from build123d import *

# Parameters (mm, degrees)
SKETCH1_W           = 177.8
SKETCH1_H           = 177.8
BOSS_EXTRUDE1_DEPTH = 12.7
SKETCH2_R           = 3.175
CUT_EXTRUDE3_DEPTH  = 13.7
SKETCH4_W           = 12.7
SKETCH4_H           = 25.4
CUT_EXTRUDE4_DEPTH  = 13.7


with BuildPart() as part:
    # Sketch1 → Boss-Extrude1 (new body)
    with BuildSketch(Plane.XY):
        with Locations((88.9, -88.9)):
            Rectangle(SKETCH1_W, SKETCH1_H)
    extrude(amount=BOSS_EXTRUDE1_DEPTH)

    # Sketch2 → Cut-Extrude3 (cut, through all)
    with BuildSketch(Plane.XY.offset(12.7)):
        with Locations((104.14, -76.2)):
            Circle(SKETCH2_R)
    extrude(amount=-CUT_EXTRUDE3_DEPTH, mode=Mode.SUBTRACT)

    # Sketch4 → Cut-Extrude4 (cut, through all)
    with BuildSketch(Plane.XY.offset(12.7)):
        with Locations((6.35, -12.7)):
            Rectangle(SKETCH4_W, SKETCH4_H)
        with Locations((6.35, -63.5)):
            Rectangle(SKETCH4_W, SKETCH4_H)
        with Locations((6.35, -114.3)):
            Rectangle(SKETCH4_W, SKETCH4_H)
        with Locations((6.35, -165.1)):
            Rectangle(SKETCH4_W, SKETCH4_H)
    extrude(amount=-CUT_EXTRUDE4_DEPTH, mode=Mode.SUBTRACT)


solid = part.part
Geometry: final body of the model. Coordinates: model frame, mm. A direction names the side the tool comes from. Coordinates: 2 decimals unless noted, no trailing zeros. Loops run counter-clockwise (first coordinate to the right, second up) from the corner with the lowest first, then second, coordinate; pieces in that order, holes last. Notation, with made-up numbers: M 49.25,71.25 L 70.25,71.25 A22 cw 70.25,98.25 Z; hole C -29,49.25 d3. An arc over 180 degrees is marked long. One line per item, written item: value. Start each with the question number.
1) Pin query (flat end, axial travel): P1, Ø4, axis at x = 5, z = 7, coming from the +Y side; P2, Ø4, axis at y = -67.5, z = 4.5, coming from the -X side; P3, Ø1.5, axis at x = 35, y = -80.5, coming from the -Z side. Return the tip coordinate at first contact, or that it passes through.
2) Cut plane C-C (y = -124). Return loops of the section in (x, z), then the cut area to 3 significant figures.
3) Cut plane A-A (x = 104.14). Return loops of the section in (y, z) (3 decimals).
4) Cut plane B-B (z = 5.75). Return loops of the section in (x, y) (3 decimals), then the cut area to 3 significant figures.
5) Draft query along Y for faces 6 (the flat face through (6, -25.4, 6)), 7 (the flat face through (6, -101.6, 6)), 8 (the flat face through (0, -38, 6)). Return one class per face: released by +Y, released by -Y, zero draft, split by the parting line, or undercut.
6) Reachability of faces 1 (the flat face through (12.7, -13, 6)), 2 (the flat face through (88, -88, 0)), 3 (the flat face through (6, -152.4, 6)), 4 (the flat face through (12.7, -114, 6)), 5 (the cylindrical face through (101.62, -78.13, 6.44)) from +Z, -Z, +X, -X, +Y, -Y: full face, straight path, thin tool, end or side. Return the list, or none.
7) Material intervals for L1, parallel to Y at x = 104.14, z = 6.75 (3 decimals); L2, parallel to X at y = -165.5, z = 11.5, sorted ascending. Write a range as from..to.
Evaluation:
1. P1: y = -25.4
1. P2: x = 12.7
1. P3: z = 0
2. outline: M 12.7,0 L 177.8,0 L 177.8,12.7 L 12.7,12.7 Z
2. area: 2,100 mm^2
3. outline: M -177.8,0 L -79.375,0 L -79.375,12.7 L -177.8,12.7 Z; M -73.025,0 L 0,0 L 0,12.7 L -73.025,12.7 Z
4. outline: M 0,-152.4 L 12.7,-152.4 L 12.7,-177.8 L 177.8,-177.8 L 177.8,0 L 12.7,0 L 12.7,-25.4 L 0,-25.4 L 0,-50.8 L 12.7,-50.8 L 12.7,-76.2 L 0,-76.2 L 0,-101.6 L 12.7,-101.6 L 12.7,-127 L 0,-127 Z; hole C 104.14,-76.2 d6.35
4. area: 30,300 mm^2
5. face 6: released by +Y
5. face 7: undercut
5. face 8: zero draft
6. face 1: +Z, -Z, -X, +Y
6. face 2: -Z, +X, -X, +Y, -Y
6. face 3: +Z, -Z, -X, -Y
6. face 4: +Z, -Z, -X
6. face 5: +Z, -Z
7. L1: -177.8..-79.375, -73.025..0
7. L2: 12.7..177.8
